```python
from build123d import *

# Parameters (mm, degrees)
SKETCH1_W                    = 1150
SKETCH1_H                    = 20
BASE_FLANGE1_DEPTH           = 1.21412
EDGE_FLANGE1_STRIP_CUT_DEPTH = 1150
EDGE_FLANGE1_DEPTH           = 1150
M8_CLEARANCE_HOLE1_D         = 9
CHAMFER1_SIZE                = 2


# Sheet-metal steps are written as plain solids
with BuildPart() as part:
    # Sketch1 → Base-Flange1 (new body)
    with BuildSketch(Plane.XY):
        Rectangle(SKETCH1_W, SKETCH1_H)
    extrude(amount=-BASE_FLANGE1_DEPTH)

    # Edge-Flange1 strip (across the edge) → Edge-Flange1 strip cut (cut)
    with BuildSketch(Plane(origin=(575, 10, 0), x_dir=(0, -0.2588190451025146, 0.96592582628907), z_dir=(-1, 0, 0))):
        Polygon((-3.043825554, 6.668712161), (-1.129475664, -0.475738894), (0.043274201, -0.161501515), (-1.87107569, 6.98294954), align=None)
    extrude(amount=EDGE_FLANGE1_STRIP_CUT_DEPTH, mode=Mode.SUBTRACT)

    # Edge-Flange1 section (across the edge) → Edge-Flange1 (add)
    with BuildSketch(Plane(origin=(575, 10, 0), x_dir=(0, -0.2588190451025146, 0.96592582628907), z_dir=(-1, 0, 0))):
        with BuildLine():
            Line((-1.21412, 0.167198672), (-1.21412, 34.84015807))
            Line((-1.21412, 34.84015807), (0, 34.84015807))
            Line((0, 34.84015807), (0, 0.167198672))
            ThreePointArc((0, 0.167198672), (0.010865026, 0.001430408), (0.043274201, -0.161501515))
            Line((0.043274201, -0.161501515), (-1.129475664, -0.475738894))
            ThreePointArc((-1.129475664, -0.475738894), (-1.192868009, -0.157044053), (-1.21412, 0.167198672))
        make_face()
    extrude(amount=EDGE_FLANGE1_DEPTH)

    # M8 Clearance Hole1 (through all)
    with Locations(Plane.XY):
        with Locations((560, 0), (400, 0), (200, 0), (0, 0), (-200, 0), (-400, 0), (-560, 0)):
            Hole(M8_CLEARANCE_HOLE1_D / 2)

    # Chamfer1
    chamfer1_edges = [part.edges().sort_by_distance(p)[0] for p in [
        (575, 43.810127161, 8.430921511),
        (-575, 43.810127161, 8.430921511),
        (575, -10, -0.60706),
        (-575, -10, -0.60706),
    ]]
    chamfer(chamfer1_edges, length=CHAMFER1_SIZE)


solid = part.part
```
Model file for the job. Use its own axes, mm. A direction names the side the tool comes from. Coordinates: 2 decimals unless noted, no trailing zeros. Loops run counter-clockwise (first coordinate to the right, second up) from the corner with the lowest first, then second, coordinate; pieces in that order, holes last. Notation, with made-up numbers: (39.5, -27) -> (49.5, -27) arc R34 cw to (49.5, 11) -> close; hole circle Ø4 at (35.5, 39.5). An arc over 180 degrees is marked (long way). Answer as a JSON object with one key per item and string values.
Q1. Cut at A-A (x = 339). List the corners of the cut face in (y, z), and give its area (3 significant figures).
Report:
{"outline": "(-10, -1.21) -> (9.83, -1.21) arc R2.48 ccw to (10.48, -1.13) -> (43.97, 7.84) -> (43.65, 9.02) -> (10.16, 0.04) arc R1.27 cw to (9.83, 0) -> (-10, 0) -> close", "area": "66.8 mm2"}
Q2. Cut at C-C (y = 20). List the corners of the cut face in (x, z).
Report:
{"outline": "(-575, 1.42) -> (575, 1.42) -> (575, 2.68) -> (-575, 2.68) -> close"}
Q3. 3-axis set-ups, long thin cutter, end or side, ignore diameter. For faces 1 (the flat face through (-8, 0, 0)), 2 (the flat face through (-8, 0, -1.214)): which of +Z, -Z, +X, -X, +Y, -Y reach the whole face in a straight line?
Report:
{"face 1": "+Z, +X, -X, -Y", "face 2": "-Z, +X, -X, +Y, -Y"}
Q4. Flat gauge pins, fed straight in: P1, Ø8, axis at x = 0, y = 0, coming from the +Z side; P2, Ø2, axis at x = 290.5, y = 29, coming from the -Z side; P3, Ø14.5, axis at x = 560, y = 0, coming from the +Z side; P4, Ø22, axis at x = -58.5, y = 4.5, coming from the +Z side. Where does each tip first touch, or does it go through?
Report:
{"P1": "passes through", "P2": "stops at z = 3.57", "P3": "stops at z = 0", "P4": "stops at z = 1.47"}
Q5. Probe probe 1 along Z at (x, y) = (-25, 10.5); probe 2 along Z at (x, y) = (86, 41.5). List the from-to ranges inside material, lowest first.
Report:
{"probe 1": "z = -1.12 to 0.13", "probe 2": "z = 7.18 to 8.44"}
Q6. Cut at B-B (z = 5.5). List the corners of the cut face in (x, y), and give its area (3 significant figures).
Report:
{"outline": "(-575, 30.53) -> (575, 30.53) -> (575, 35.22) -> (-575, 35.22) -> close", "area": "5,390 mm2"}
